Could you check a few things on this model? Use its own coordinates, in mm. A direction names the side the tool comes from. Round coordinates to 2 decimals unless told otherwise and drop trailing zeros. Loops run counter-clockwise (first coordinate to the right, second up) from the corner with the lowest first, then second, coordinate; pieces in that order, holes last. Notation, with made-up numbers: (30.25, 39) - (83.25, 39) arc R6 cw to (83.25, 43) - close; hole circle Ø10 at (-29, 74.25). An arc over 180 degrees is marked (long way). Put each result on its own line as item: value. Start each with the question number.
from build123d import *

# Parameters (mm, degrees)
SKETCH_1_R      = 1.5
SKETCH_1_R_2    = 8
EXTRUDE_1_DEPTH = 4


with BuildPart() as part:
    # 草图1 → 凸台-拉伸1 (new body)
    with BuildSketch(Plane(origin=(0, 0, 0), x_dir=(0, 0, -1), z_dir=(1, 0, 0))):
        with BuildLine():
            Line((20.589035366, 12), (26.5, 12))
            ThreePointArc((26.5, 12), (27.560660172, 11.560660172), (28, 10.5))
            Line((28, 10.5), (28, -10.5))
            ThreePointArc((28, -10.5), (27.560660172, -11.560660172), (26.5, -12))
            Line((26.5, -12), (-26.5, -12))
            ThreePointArc((-26.5, -12), (-27.560660172, -11.560660172), (-28, -10.5))
            Line((-28, -10.5), (-28, 10.5))
            ThreePointArc((-28, 10.5), (-27.560660172, 11.560660172), (-26.5, 12))
            Line((-26.5, 12), (-10.589035366, 12))
            ThreePointArc((-10.589035366, 12), (-10.040758683, 12.103793469), (-9.568358717, 12.400809763))
            Line((-9.568358717, 12.400809763), (-3.431641283, 18.099190237))
            ThreePointArc((-3.431641283, 18.099190237), (-2.959241317, 18.396206531), (-2.410964634, 18.5))
            Line((-2.410964634, 18.5), (12.410964634, 18.5))
            ThreePointArc((12.410964634, 18.5), (12.959241317, 18.396206531), (13.431641283, 18.099190237))
            Line((13.431641283, 18.099190237), (19.568358717, 12.400809763))
            ThreePointArc((19.568358717, 12.400809763), (20.040758683, 12.103793469), (20.589035366, 12))
        make_face()
        with Locations((0, 15)):
            Circle(SKETCH_1_R, mode=Mode.SUBTRACT)
        with Locations((20, 0)):
            Circle(SKETCH_1_R, mode=Mode.SUBTRACT)
        with Locations((-10, 0)):
            Circle(SKETCH_1_R_2, mode=Mode.SUBTRACT)
        with Locations((24.5, 5)):
            Circle(SKETCH_1_R, mode=Mode.SUBTRACT)
        with Locations((24.5, -5)):
            Circle(SKETCH_1_R, mode=Mode.SUBTRACT)
        with Locations((-24.5, 5)):
            Circle(SKETCH_1_R, mode=Mode.SUBTRACT)
        with Locations((-24.5, -5)):
            Circle(SKETCH_1_R, mode=Mode.SUBTRACT)
        with Locations((10, 15)):
            Circle(SKETCH_1_R, mode=Mode.SUBTRACT)
    extrude(amount=EXTRUDE_1_DEPTH)


solid = part.part
Item 1: Suppose I cut it at B-B, the plane x = 2.2. Count the separate pieces of the cut face and the enclosed holes in it, then the cut area to 3 significant figures.
Item 2: Suppose I cut it at C-C, the plane y = 15. List the corners of the cut face in (x, z) for me, then the cut area to 3 significant figures.
Item 3: Will these pins go through, and if not, where does the flat tip stop? P1, Ø3.5, axis at y = 0, z = -20, coming from the -X side; P2, Ø1.2, axis at x = 2, z = 18, coming from the +Y side; P3, Ø2.5, axis at y = 15, z = 0, coming from the +X side.
Item 4: I need wall thicknesses on line 1 (Y direction, x = 3, z = -10); line 2 (Y direction, x = 2.2, z = 24.5); line 3 (Y direction, x = 3.75, z = -19). Which ranges of each line are inside material? Lowest first, please. Write a range as from..to.
Item 5: On a 3-axis mill with a long thin cutter (end or side, diameter ignored), from which of +Z, -Z, +X, -X, +Y, -Y can I reach the whole of each face in a straight line? I mean faces 1 (the face through (1.97, -7.81, 11.73)), 2 (the face through (2, 12, -24)). Say none if no direction works.
Item 6: Suppose I cut it at A-A, the plane z = -10. List the corners of the cut face in (x, y) for me, then the cut area to 3 significant figures.
Item 7: Suppose I cut it at D-D, the plane z = 7.5. List the corners of the cut face in (x, y) for me, then the cut area to 3 significant figures.
Item 8: Thinking about a two-plate mould opening in Z: for faces 3 (the face through (1.97, -11.57, 27.55)), 4 (the face through (1.97, 18.4, -12.95)), 5 (the face through (2, -5, -23)), which applies, released by +Z, released by -Z, zero draft, split by the parting line, or undercut?
Numbers:
1. separate pieces: 1
1. enclosed holes: 8
1. area: 1,240 mm^2
2. outline: (0, -16.77) - (4, -16.77) - (4, -11.5) - (0, -11.5) - close; (0, -8.5) - (4, -8.5) - (4, -1.5) - (0, -1.5) - close; (0, 1.5) - (4, 1.5) - (4, 6.77) - (0, 6.77) - close
2. area: 70.2 mm^2
3. P1: x = 0
3. P2: y = 12
3. P3: through
4. line 1: -12..13.5, 16.5..18.5
4. line 2: -12..-6.5, -3.5..3.5, 6.5..12
4. line 3: -12..-1.12, 1.12..12.93
5. face 1: +X, -X
5. face 2: -Z, +X, -X, +Y
6. outline: (0, -12) - (4, -12) - (4, 13.5) - (0, 13.5) - close; (0, 16.5) - (4, 16.5) - (4, 18.5) - (0, 18.5) - close
6. area: 110 mm^2
7. outline: (0, -12) - (4, -12) - (4, -7.6) - (0, -7.6) - close; (0, 7.6) - (4, 7.6) - (4, 14.32) - (0, 14.32) - close
7. area: 44.5 mm^2
8. face 3: released by +Z
8. face 4: released by -Z
8. face 5: undercut
